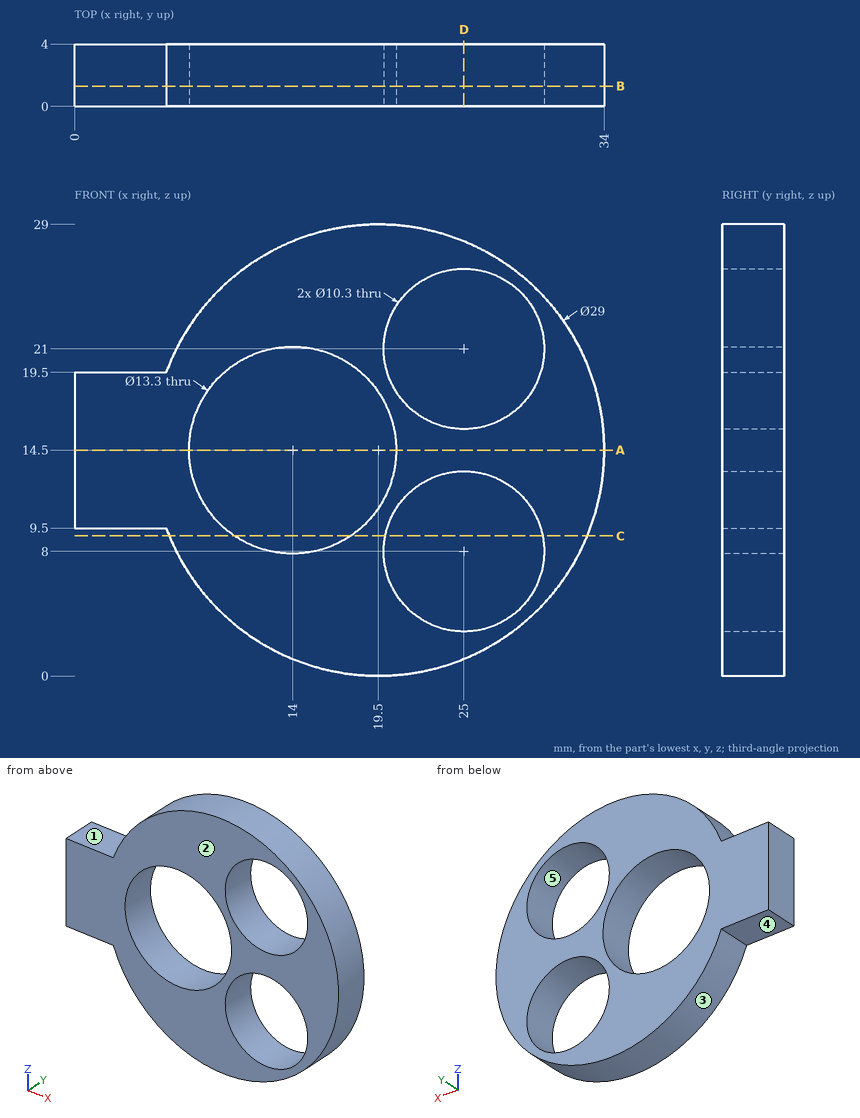
Answer from the drawing. Dimensions are ordinates in mm from the lowest x, y and z of the part. A direction names the side the tool comes from. Give positions to 0.01 mm unless a question says otherwise; leave off trailing zeros. Order: outer loops, then holes, each group sorted by start corner. A loop starts at its lowest first (then second) coordinate and runs counter-clockwise, first axis right, second up.
Item 1: Which of the six approach directions +Z, -Z, +X, -X, +Y, -Y give full straight-line access (tool end or side, diameter ignored) to the marked faces 1 and 2?
From the geometry:
face 1: +Z, -X, +Y, -Y
face 2: +Z, -Z, +X, -X, -Y
Item 2: The part is cut by section B-B, the plane y = 1.3. Give the vertices of the cut face in (x, z).
From the geometry:
outline: (0, 9.5) - (5.89, 9.5) arc R14.5 ccw (long way) to (5.89, 19.5) - (0, 19.5) - close; hole circle Ø13.3 at (14, 14.5); hole circle Ø10.3 at (25, 8); hole circle Ø10.3 at (25, 21)
Item 3: Given pin 1 Ø1.2 at (x, y) = (4, 2) entering from +Z; pin 2 Ø1.5 at (x, y) = (10.5, 3) entering from -Z, each flat-ended and moving along its own axis, determine where each tip first touches the part or whether it passes through.
From the geometry:
pin 1: stops at z = 19.5
pin 2: stops at z = 2.58
Item 4: The part is cut by section A-A, the plane z = 14.5. Give the vertices of the cut face in (x, y), and give its area (3 significant figures).
From the geometry:
outline: (0, 0) - (7.35, 0) - (7.35, 4) - (0, 4) - close; (20.65, 0) - (34, 0) - (34, 4) - (20.65, 4) - close
area: 82.8 mm2
Item 5: For a pull along Z with two mould halves and no side action, classify the marked faces 3, 4 and 5 as pulls with the +Z half, pulls with the -Z half, needs draft (parallel to the pull), parting line crosses it, or undercut.
From the geometry:
face 3: parting line crosses it
face 4: pulls with the -Z half
face 5: undercut
Item 6: The part is cut by section D-D, the plane x = 25. Give the vertices of the cut face in (y, z), and give its area (3 significant figures).
From the geometry:
outline: (0, 1.08) - (4, 1.08) - (4, 2.85) - (0, 2.85) - close; (0, 13.15) - (4, 13.15) - (4, 15.85) - (0, 15.85) - close; (0, 26.15) - (4, 26.15) - (4, 27.92) - (0, 27.92) - close
area: 24.9 mm2
Item 7: The part is cut by section C-C, the plane z = 9. Give the vertices of the cut face in (x, y), and give its area (3 significant figures).
From the geometry:
outline: (6.08, 0) - (10.26, 0) - (10.26, 4) - (6.08, 4) - close; (17.74, 0) - (19.95, 0) - (19.95, 4) - (17.74, 4) - close; (30.05, 0) - (32.92, 0) - (32.92, 4) - (30.05, 4) - close
area: 37.0 mm2
Item 8: Find the intervals of material crossed by probe 1 along X at (y, z) = (1.5, 19.25); probe 2 along X at (y, z) = (1.75, 14.5); probe 3 along Z at (x, y) = (28, 2.65), in increasing order.
From the geometry:
probe 1: x = 0 to 9.35, 18.65 to 20.16, 29.84 to 33.2
probe 2: x = 0 to 7.35, 20.65 to 34
probe 3: z = 2.75 to 3.81, 12.19 to 16.81, 25.19 to 26.25
